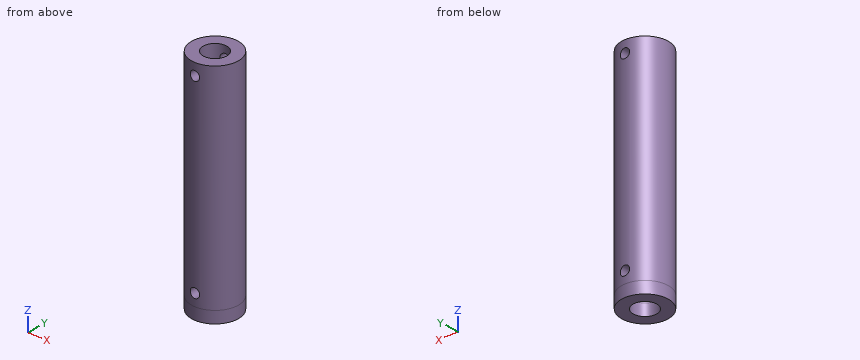
Autodesk Inventor part; units mm, degrees
ref_plane "YZ Plane" through (0, 0, 0) normal (1, 0, 0) x (0, 1, 0)
ref_plane "XZ Plane" through (0, 0, 0) normal (0, 1, 0) x (-1, 0, 0)
ref_plane "XY Plane" through (0, 0, 0) normal (0, 0, 1) x (1, 0, 0)
sketch "Esquisse1" plane through (0, 0, 0) normal (0, 0, 1) x (1, 0, 0)
  circle A0 centre (0, 0) radius 9.9
  circle A1 centre (0, 0) radius 5
  dimension "d0" = 19.8
  dimension "d1" = 10
extrude "Extrusion1" add sketch "Esquisse1" along normal blind 90
sketch "Esquisse2" plane through (0, 0, 0) normal (0, 1, 0) x (-1, 0, 0)
  line L0 (0, 0) -> (0, 5)
  line L1 (9.9, 90) -> (-9.9, 90)
  line L2 (0, 90) -> (0, 85)
  dimension "d4" = 5
  dimension "d5" = 5
hole "Perçage1" at (0, 0, 5) at (0, 0, 85) direction (0, -1, 0) diameter 4 end through all both
sketch "Esquisse3" plane through (0, 0, 0) normal (0, 0, -1) x (-1, 0, 0)
  circle A0 centre (0, 0) radius 5
  circle A1 centre (0, 0) radius 9.9
extrude "Extrusion2" add sketch "Esquisse3" along normal blind 5
properties part number "tubelong_rocker"
The model under review builds one solid part; all positions refer to its coordinate system, in mm. Give positions to 0.01 mm unless a question says otherwise; leave off trailing zeros. Write each loop counter-clockwise with the first axis right and the second up, starting at its lowest first coordinate (ties: lowest second). Pieces come first, ordered by that corner, then holes. Notation, with made-up numbers: M -36.75,17.25 L 8.25,17.25 A25 cw 8.25,40.25 Z; hole C -33.5,6.5 d8. An arc over 180 degrees is marked long. Write item = value, one per line. Start each with the question number.
Q1. We need section A-A (y = 0). State the section outline as (x, z) points, plus the area to 3 significant figures.
Q2. For line 1 (Z direction, x = 0.25, y = 9); line 2 (Y direction, x = 0, z = -1.95), list the stretches that pass through material, from the lowest coordinate up.
Q3. We need section C-C (z = 85). State the section outline as (x, y) points.
Q4. We need section B-B (x = 0). State the section outline as (y, z) points, plus the area to 3 significant figures.
Q5. Clearance check with flat-ended pins moving along their axes: pin 1 (2 mm diameter, centred on y = -4.5, z = 27.5, fed in from +X); pin 2 (3 mm diameter, centred on y = 3.5, z = 40.5, fed in from -X). State where each tip first meets the part, or that it passes through.
Q6. We need section D-D (z = 17). State the section outline as (x, y) points, plus the area to 3 significant figures.
Result set:
q1.outline = M -9.9,-5 L -5,-5 L -5,90 L -9.9,90 Z; M 5,-5 L 9.9,-5 L 9.9,90 L 5,90 Z
q1.area = 931 mm2
q2.line_1 = -5 to 3.02, 6.98 to 83.02, 86.98 to 90
q2.line_2 = -9.9 to -5, 5 to 9.9
q3.outline = M -2,-9.7 L -2,-4.58 A5 cw -2,4.58 L -2,9.7 A9.9 ccw Z; M 2,-9.7 A9.9 ccw 2,9.7 L 2,4.58 A5 cw 2,-4.58 Z
q4.outline = M -9.9,-5 L -5,-5 L -5,3 L -9.9,3 Z; M -9.9,7 L -5,7 L -5,83 L -9.9,83 Z; M -9.9,87 L -5,87 L -5,90 L -9.9,90 Z; M 5,-5 L 9.9,-5 L 9.9,3 L 5,3 Z; M 5,7 L 9.9,7 L 9.9,83 L 5,83 Z; M 5,87 L 9.9,87 L 9.9,90 L 5,90 Z
q4.area = 853 mm2
q5.pin_1 = 9.26
q5.pin_2 = -9.7
q6.outline = C 0,0 d19.8; hole C 0,0 d10
q6.area = 229 mm2
